Work out the finished part from the listing and answer in its coordinate system (mm). Face numbers are marked on the shaded views. A direction names the side the tool comes from. Give positions to 0.01 mm unless a question says otherwise; leave off trailing zeros. Write each loop counter-clockwise with the first axis right and the second up, starting at its lowest first coordinate (ties: lowest second). Pieces come first, ordered by that corner, then holes.
1) Given pin 1 Ø6 at (y, z) = (8, 6.5) entering from +X; pin 2 Ø6.5 at (x, z) = (-15, 0) entering from -Y; pin 3 Ø6 at (x, z) = (6, -7) entering from -Y; pin 4 Ø5 at (x, z) = (0, 0) entering from -Y, each flat-ended and moving along its own axis, determine where each tip first touches the part or whether it passes through.
2) Straight lines are drawn through the part: probe 1 along X at (y, z) = (0.6, 0); probe 2 along X at (y, z) = (3.85, 0); probe 3 along Z at (x, y) = (0, 20.75). For each, find the intervals that lie inside material, in ascending order.
3) Determine the mould class of the marked faces 4, 5 and 6 for opening direction Z: pulls with the +Z half, pulls with the -Z half, needs draft (parallel to the pull), parting line crosses it, or undercut.
4) Find section D-D (y = 19.75). Determine the outline of the cut face in (x, z), plus the area to 3 significant figures.
5) A tool of negligible diameter and unlimited length cuts with its end or side. For the marked faces 1, 2 and 3, from which of +Z, -Z, +X, -X, +Y, -Y can it reach the whole face along a straight path? Write none if from no direction.
6) Find section A-A (x = 0). Determine the outline of the cut face in (y, z).
7) Find section C-C (y = 1.5). Count the separate pieces of the cut face and the enclosed holes in it, plus the area to 3 significant figures.
```python
from build123d import *

# Parameters (mm, degrees)
ESQUISSE1_W             = 10
ESQUISSE1_H             = 20
BOSS_EXTRU_1_DEPTH      = 15
BOSS_EXTRU_1_2_DEPTH    = 15
ESQUISSE3_W             = 40
ESQUISSE3_H             = 20
BOSS_EXTRU_2_DEPTH      = 8
ESQUISSE4_R             = 3.2
ENL_V_MAT_EXTRU_1_DEPTH = 10
ESQUISSE1_3_R           = 2.75
ENL_V_MAT_EXTRU_3_DEPTH = 7
ESQUISSE1_4_R           = 3.5
ESQUISSE1_4_R_2         = 2.75
ENL_V_MAT_EXTRU_4_DEPTH = 1
CHANFREIN1_SIZE         = 3
CONG_1_R                = 3


with BuildPart() as part:
    # Esquisse1 → Boss.-Extru.1 (new body)
    with BuildSketch(Plane(origin=(0, 0, 0), x_dir=(1, 0, 0), z_dir=(0, 1, 0))):
        with Locations((-15, 0)):
            Rectangle(ESQUISSE1_W, ESQUISSE1_H)
    extrude(amount=BOSS_EXTRU_1_DEPTH)



with BuildPart() as body_2:
    # Esquisse1 → Boss.-Extru.1 2 (new body)
    with BuildSketch(Plane(origin=(0, 0, 0), x_dir=(1, 0, 0), z_dir=(0, 1, 0))):
        with Locations((15, 0)):
            Rectangle(ESQUISSE1_W, ESQUISSE1_H)
    extrude(amount=BOSS_EXTRU_1_2_DEPTH)


with BuildPart() as part_1:
    add(part.part)

    add(body_2.part)  # Boss.-Extru.2 merges body 2
    # Esquisse3 → Boss.-Extru.2 (add)
    with BuildSketch(Plane(origin=(0, 15, 0), x_dir=(1, 0, 0), z_dir=(0, 1, 0))):
        Rectangle(ESQUISSE3_W, ESQUISSE3_H)
    extrude(amount=BOSS_EXTRU_2_DEPTH)

    # Esquisse4 → Enl_v. mat.-Extru.1 (cut)
    with BuildSketch(Plane(origin=(0, 23, 0), x_dir=(1, 0, 0), z_dir=(0, 1, 0))):
        Circle(ESQUISSE4_R)
    extrude(amount=-ENL_V_MAT_EXTRU_1_DEPTH, mode=Mode.SUBTRACT)

    # Esquisse1_3 → Enl_v. mat.-Extru.3 (cut)
    with BuildSketch(Plane(origin=(0, 0, 0), x_dir=(1, 0, 0), z_dir=(0, 1, 0))):
        with Locations((-15, 0)):
            Circle(ESQUISSE1_3_R)
        with Locations((15, 0)):
            Circle(ESQUISSE1_3_R)
    extrude(amount=ENL_V_MAT_EXTRU_3_DEPTH, mode=Mode.SUBTRACT)

    # Esquisse1_4 → Enl_v. mat.-Extru.4 (cut)
    with BuildSketch(Plane(origin=(0, 0, 0), x_dir=(1, 0, 0), z_dir=(0, 1, 0))):
        with Locations((-15, 0)):
            Circle(ESQUISSE1_4_R)
        with Locations((-15, 0)):
            Circle(ESQUISSE1_4_R_2, mode=Mode.SUBTRACT)
        with Locations((15, 0)):
            Circle(ESQUISSE1_4_R)
        with Locations((15, 0)):
            Circle(ESQUISSE1_4_R_2, mode=Mode.SUBTRACT)
    extrude(amount=ENL_V_MAT_EXTRU_4_DEPTH, mode=Mode.SUBTRACT)

    # Chanfrein1
    chanfrein1_edges = [part_1.edges().sort_by_distance(p)[0] for p in [
        (20, 11.5, 10),
        (20, 11.5, -10),
        (10, 7.5, -10),
        (10, 7.5, 10),
        (-20, 11.5, 10),
        (-20, 11.5, -10),
        (-10, 7.5, -10),
        (-10, 7.5, 10),
    ]]
    chamfer(chanfrein1_edges, length=CHANFREIN1_SIZE)

    # Cong_1
    cong_1_edges = [part_1.edges().sort_by_distance(p)[0] for p in [
        (-10, 7.5, -7),
        (-20, 11.5, 7),
        (-20, 11.5, -7),
        (10, 7.5, 7),
        (10, 7.5, -7),
        (-17, 11.5, -10),
        (-13, 7.5, -10),
        (17, 11.5, -10),
        (13, 7.5, -10),
        (20, 11.5, 7),
        (20, 11.5, -7),
        (-17, 11.5, 10),
        (17, 11.5, 10),
        (-13, 7.5, 10),
        (13, 7.5, 10),
        (-10, 7.5, 7),
    ]]
    fillet(cong_1_edges, radius=CONG_1_R)


solid = part_1.part
```
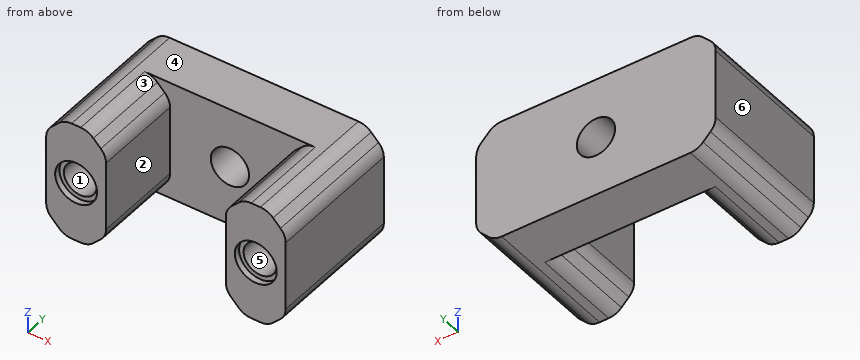
Results:
1. pin 1: stops at x = 20
1. pin 2: stops at y = 1
1. pin 3: stops at y = 15
1. pin 4: passes through
2. probe 1: x = -20 to -18.5, -11.5 to -10, 10 to 11.5, 18.5 to 20
2. probe 2: x = -20 to -17.75, -12.25 to -10, 10 to 12.25, 17.75 to 20
2. probe 3: z = -10 to -3.2, 3.2 to 10
3. face 4: pulls with the +Z half
3. face 5: undercut
3. face 6: needs draft
4. outline: (-20, -5.76) arc R3 ccw to (-19.12, -7.88) - (-17.88, -9.12) arc R3 ccw to (-15.76, -10) - (15.76, -10) arc R3 ccw to (17.88, -9.12) - (19.12, -7.88) arc R3 ccw to (20, -5.76) - (20, 5.76) arc R3 ccw to (19.12, 7.88) - (17.88, 9.12) arc R3 ccw to (15.76, 10) - (-15.76, 10) arc R3 ccw to (-17.88, 9.12) - (-19.12, 7.88) arc R3 ccw to (-20, 5.76) - close; hole circle Ø6.4 at (0, 0)
4. area: 748 mm2
5. face 1: -Y
5. face 2: +Z, -Z, -Y
5. face 3: +Z, -Y
6. outline: (15, -10) - (23, -10) - (23, -3.2) - (15, -3.2) - close; (15, 3.2) - (23, 3.2) - (23, 10) - (15, 10) - close
7. separate pieces: 2
7. enclosed holes: 2
7. area: 313 mm2
